from build123d import *

# Parameters (mm, degrees)
F0_W        = 260
F0_H        = 26
F0_R        = 2.7
F0_R_2      = 2
F1_DEPTH    = 4
F2_W        = 260
F2_H        = 4
F3_DEPTH    = 10
F4_SIZE     = 10
F5_T1_DEPTH = 29


# Not quite as in the source:
# - a fillet or chamfer that OpenCascade refuses, or shapes differently, is made with other operations: its cross-section is extruded or revolved along the edge and cut away or added


with BuildPart() as f1:
    # F0 (on Top) → F1 (new body)
    with BuildSketch(Plane.XY):
        Rectangle(F0_W, F0_H)
        with Locations((-120, 0)):
            Circle(F0_R, mode=Mode.SUBTRACT)
        with Locations((-35.75, 5)):
            Circle(F0_R_2, mode=Mode.SUBTRACT)
        with Locations((35.75, 5)):
            Circle(F0_R_2, mode=Mode.SUBTRACT)
        with Locations((120, 0)):
            Circle(F0_R, mode=Mode.SUBTRACT)
    extrude(amount=F1_DEPTH)

    # F2 (on face) → F3 (join)
    with BuildSketch(Plane.XY.offset(4)):
        with Locations((0, -11)):
            Rectangle(F2_W, F2_H)
    extrude(amount=F3_DEPTH)

    # F4
    f4_edges = [f1.edges().sort_by_distance(p)[0] for p in [
        (-130, -11, 14),
        (130, -11, 14),
    ]]
    chamfer(f4_edges, length=F4_SIZE)

    # F5: fillet of radius 5 on 4 edges, made by hand

    # F5_s2 → F5_t1 (cut)
    with BuildSketch(Plane.XY.offset(-12.5)):
        with BuildLine():
            ThreePointArc((125, 13), (128.5355339059, 11.5355339059), (130, 8))
            Line((130, 8), (130, 13))
            Line((130, 13), (125, 13))
        make_face()
        with BuildLine():
            ThreePointArc((125, -13), (128.5355339059, -11.5355339059), (130, -8))
            Line((130, -8), (130, -13))
            Line((130, -13), (125, -13))
        make_face()
        with BuildLine():
            ThreePointArc((-130, 8), (-128.5355339059, 11.5355339059), (-125, 13))
            Line((-125, 13), (-130, 13))
            Line((-130, 13), (-130, 8))
        make_face()
        with BuildLine():
            ThreePointArc((-130, -8), (-128.5355339059, -11.5355339059), (-125, -13))
            Line((-125, -13), (-130, -13))
            Line((-130, -13), (-130, -8))
        make_face()
    extrude(amount=F5_T1_DEPTH, mode=Mode.SUBTRACT)


solid = f1.part
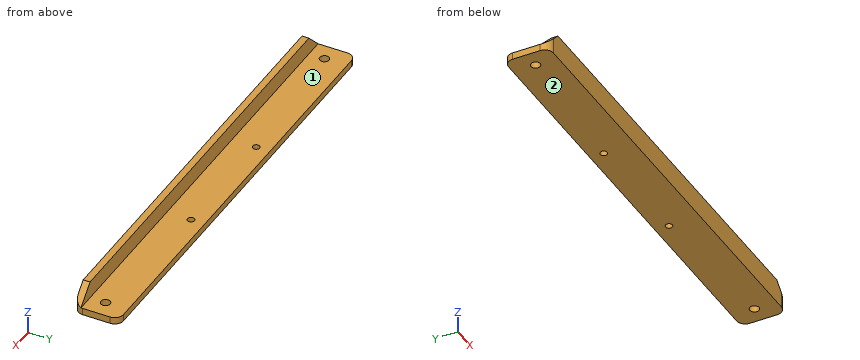
The listing builds one solid part. Answer for the finished solid, in the listing's coordinates (mm). Face numbers are marked on the shaded views. A direction names the side the tool comes from. Give positions to 0.01 mm unless a question says otherwise; leave off trailing zeros. Write each loop counter-clockwise with the first axis right and the second up, starting at its lowest first coordinate (ties: lowest second). Pieces come first, ordered by that corner, then holes. Notation, with made-up numbers: (41, 56.5) - (69, 56.5) arc R22 ccw to (69, 90.5) - close; hole circle Ø5 at (15.25, 11). An arc over 180 degrees is marked (long way). One line per question, with ' | ' between items. Start each with the question number.
1. Given P1, Ø6, axis at x = -120, y = 0, coming from the +Z side; P2, Ø2, axis at x = -94, z = 12, coming from the +Y side; P3, Ø8, axis at x = -69.5, y = -8, coming from the -Z side, each flat-ended and moving along its own axis, determine where each tip first touches the part or whether it passes through.
2. For the marked faces 1 and 2, determine the directions among +Z, -Z, +X, -X, +Y, -Y from which every point of the face is accessible in a straight line to the end or side of a thin tool.
3. Section B-B, the plane x = -100 is taken. Determine the outline of the cut face in (y, z), then the cut area to 3 significant figures.
4. Section C-C, the plane z = 11.25 is taken. Determine the outline of the cut face in (x, y), then the cut area to 3 significant figures.
5. Straight lines are drawn through the part: line 1 (Y direction, x = -35.75, z = 0.9); line 2 (Y direction, x = 120, z = 1.75); line 3 (Z direction, x = -78, y = -3). For each, find the intervals that lie inside material, in ascending order.
6. Section A-A, the plane y = 0 is taken. Determine the outline of the cut face in (x, z).
Result:
1) P1: stops at z = 4 | P2: stops at y = -9 | P3: stops at z = 0
2) face 1: +Z, +X, -X, +Y | face 2: -Z, +X, -X, +Y, -Y
3) outline: (-13, 0) - (13, 0) - (13, 4) - (-9, 4) - (-9, 14) - (-13, 14) - close | area: 144 mm2
4) outline: (-122.75, -13) - (122.75, -13) - (122.75, -9) - (-122.75, -9) - close | area: 982 mm2
5) line 1: y = -13 to 3, 7 to 13 | line 2: y = -13 to -2.7, 2.7 to 13 | line 3: z = 0 to 4
6) outline: (-130, 0) - (-122.7, 0) - (-122.7, 4) - (-130, 4) - close; (-117.3, 0) - (117.3, 0) - (117.3, 4) - (-117.3, 4) - close; (122.7, 0) - (130, 0) - (130, 4) - (122.7, 4) - close
